Read the model definition and answer for the solid it produces. Units are mm, in the model's axes. A direction names the side the tool comes from. Round coordinates to 2 decimals unless told otherwise and drop trailing zeros. Order: outer loops, then holes, each group sorted by start corner. A loop starts at its lowest first (then second) coordinate and runs counter-clockwise, first axis right, second up.
from build123d import *

# Parameters (mm, degrees)
F0_R     = 41.275
F0_R_2   = 38.1
F2_DEPTH = 13.335
F3_DEPTH = 6.985


with BuildPart() as f2:
    # F0 (on Top) → F2 (new body)
    with BuildSketch(Plane.XY):
        Circle(F0_R)
        Circle(F0_R_2, mode=Mode.SUBTRACT)
    extrude(amount=F2_DEPTH)

    # F1 (on face) → F3 (join)
    with BuildSketch(Plane.XY):
        with BuildLine():
            ThreePointArc((-26.9875, 26.8939555244), (-27.7941461706, 26.0594596768), (-28.575, 25.2007812379))
            Line((-28.575, 25.2007812379), (-28.575, -25.2007812379))
            ThreePointArc((-28.575, -25.2007812379), (-27.7941461706, -26.0594596768), (-26.9875, -26.8939555244))
            Line((-26.9875, -26.8939555244), (-26.9875, 26.8939555244))
        make_face()
        with BuildLine():
            ThreePointArc((26.8939555244, 26.9875), (26.0594596768, 27.7941461706), (25.2007812379, 28.575))
            Line((25.2007812379, 28.575), (-25.2007812379, 28.575))
            ThreePointArc((-25.2007812379, 28.575), (-26.0594596768, 27.7941461706), (-26.8939555244, 26.9875))
            Line((-26.8939555244, 26.9875), (26.8939555244, 26.9875))
        make_face()
        with BuildLine():
            Line((28.575, -25.2007812379), (28.575, 25.2007812379))
            ThreePointArc((28.575, 25.2007812379), (27.7941461706, 26.0594596768), (26.9875, 26.8939555244))
            Line((26.9875, 26.8939555244), (26.9875, -26.8939555244))
            ThreePointArc((26.9875, -26.8939555244), (27.7941461706, -26.0594596768), (28.575, -25.2007812379))
        make_face()
        with BuildLine():
            Line((-25.2007812379, -28.575), (25.2007812379, -28.575))
            ThreePointArc((25.2007812379, -28.575), (26.0594596768, -27.7941461706), (26.8939555244, -26.9875))
            Line((26.8939555244, -26.9875), (-26.8939555244, -26.9875))
            ThreePointArc((-26.8939555244, -26.9875), (-26.0594596768, -27.7941461706), (-25.2007812379, -28.575))
        make_face()
        with BuildLine():
            Line((-25.2007812379, 28.575), (25.2007812379, 28.575))
            ThreePointArc((25.2007812379, 28.575), (0, 38.1), (-25.2007812379, 28.575))
        make_face()
        with BuildLine():
            Line((-28.575, -25.2007812379), (-28.575, 25.2007812379))
            ThreePointArc((-28.575, 25.2007812379), (-38.1, 0), (-28.575, -25.2007812379))
        make_face()
        with BuildLine():
            ThreePointArc((-25.2007812379, -28.575), (0, -38.1), (25.2007812379, -28.575))
            Line((25.2007812379, -28.575), (-25.2007812379, -28.575))
        make_face()
        with BuildLine():
            ThreePointArc((38.1, 0), (35.639286609, 13.4703841816), (28.575, 25.2007812379))
            Line((28.575, 25.2007812379), (28.575, -25.2007812379))
            ThreePointArc((28.575, -25.2007812379), (35.639286609, -13.4703841816), (38.1, 0))
        make_face()
    extrude(amount=F3_DEPTH)


solid = f2.part
Q1. Straight lines are drawn through the part: probe 1 along Y at (x, z) = (0, 3.25) (1 decimal); probe 2 along Y at (x, z) = (0, 10.75) (3 decimals); probe 3 along Z at (x, y) = (-4.5, -33) (3 decimals). For each, find the intervals that lie inside material, in ascending order.
Outcome:
probe 1: y = -41.3 to -27, 27 to 41.3
probe 2: y = -41.275 to -38.1, 38.1 to 41.275
probe 3: z = 0 to 6.985
Q2. A cutting plane is placed at A-A, the plane y = 0. Give the vertices of the cut face in (x, z) (1 decimal), plus the area to 3 significant figures.
Outcome:
outline: (-41.3, 0) - (-27, 0) - (-27, 7) - (-38.1, 7) - (-38.1, 13.3) - (-41.3, 13.3) - close; (27, 0) - (41.3, 0) - (41.3, 13.3) - (38.1, 13.3) - (38.1, 7) - (27, 7) - close
area: 240 mm2
Q3. A cutting plane is placed at D-D, the plane x = 32. Give the vertices of the cut face in (y, z) (3 decimals).
Outcome:
outline: (-26.07, 0) - (26.07, 0) - (26.07, 13.335) - (20.679, 13.335) - (20.679, 6.985) - (-20.679, 6.985) - (-20.679, 13.335) - (-26.07, 13.335) - close
Q4. For faces 1 (the face through (12, -36.5, 13.335)), 2 (the face through (-26.988, 0, 3)), 3 (the face through (0, -31, 6.985)), determine the directions among +Z, -Z, +X, -X, +Y, -Y from which every point of the face is accessible in a straight line to the end or side of a thin tool.
Outcome:
face 1: +Z, +X, -X, +Y, -Y
face 2: +Z, -Z
face 3: +Z
Q5. Flat-ended cylindrical pins translate along their axes: pin 1 (3.5 mm diameter, centred on x = -34, y = 5.5, fed in from +Z) (3 decimals); pin 2 (3.5 mm diameter, centred on x = 2.5, z = 2, fed in from +Y); pin 3 (5.5 mm diameter, centred on y = 4.5, z = 2.5, fed in from +X). Find the tip coordinate at first contact, or state that the pin passes through.
Outcome:
pin 1: stops at z = 6.985
pin 2: stops at y = 41.27
pin 3: stops at x = 41.24
